Geometry check sheet. Reference: the model listing, model coordinates, mm. Face numbers are marked on the shaded views. A direction names the side the tool comes from. Give positions to 0.01 mm unless a question says otherwise; leave off trailing zeros. Loops run counter-clockwise (first coordinate to the right, second up) from the corner with the lowest first, then second, coordinate; pieces in that order, holes last. Notation, with made-up numbers: (48.5, 48.5) -> (57.5, 48.5) arc R13 cw to (57.5, 69.5) -> close; hole circle Ø1 at (75.5, 88.25). An arc over 180 degrees is marked (long way). Answer as a JSON object with one key per item and string values.
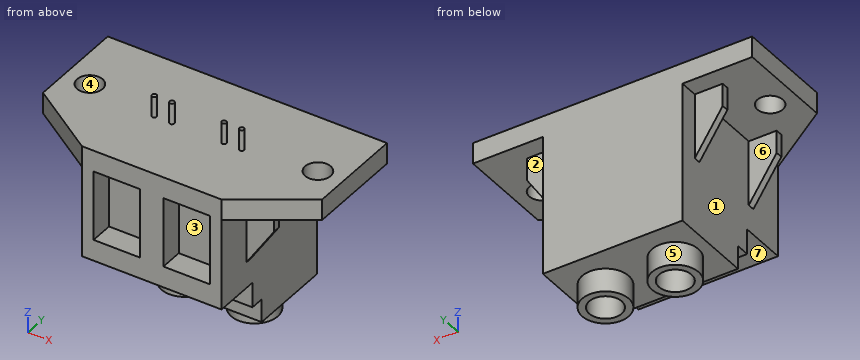
from build123d import *

# Parameters (mm, degrees)
SKETCH_1_R           = 2.75
EXTRUDE_1_DEPTH      = 4.5
EXTRUDE_2_DEPTH      = 15
EXTRUDE_2_DEPTH_BACK = 15
SKETCH_3_R           = 5
SKETCH_3_R_2         = 3.5
EXTRUDE_3_DEPTH      = 5
SKETCH_4_W           = 10
SKETCH_4_H           = 15
CUT_EXTRUDE_1_DEPTH  = 5
SKETCH_5_R           = 0.5
EXTRUDE_4_DEPTH      = 4.5
SKETCH_6_W           = 6
SKETCH_6_H           = 1.5
EXTRUDE_5_DEPTH      = 14
CUT_EXTRUDE_2_DEPTH  = 20


with BuildPart() as part:
    # Эскиз1 → Вытянуть1 (new body)
    with BuildSketch(Plane.XY):
        Polygon((-15, -16.9), (-30, -6.9), (-30, 14.1), (30, 14.1), (30, -6.9), (15, -16.9), align=None)
        with Locations((-24.5, 0)):
            Circle(SKETCH_1_R, mode=Mode.SUBTRACT)
        with Locations((24.5, 0)):
            Circle(SKETCH_1_R, mode=Mode.SUBTRACT)
    extrude(amount=EXTRUDE_1_DEPTH)

    # Эскиз2 → Вытянуть2 (add, two sides: drawn at the far end of the back side and taken through both)
    with BuildSketch(Plane(origin=(0, 0, 0), x_dir=(0, 0, -1), z_dir=(1, 0, 0)).offset(-EXTRUDE_2_DEPTH_BACK)):
        Polygon((0, -16.9), (19.60451018, -16.9), (19.60451018, -6.9), (25, -6.9), (25, -3.9), (30, -3.9), (30, 14.1), (0, 14.1), align=None)
    extrude(amount=EXTRUDE_2_DEPTH + EXTRUDE_2_DEPTH_BACK)

    # Эскиз3 → Вытянуть3 (add)
    # profile 1 of 2: a face of its own
    with BuildSketch(Plane(origin=(0, 0, -30), x_dir=(-1, 0, 0), z_dir=(0, 0, -1))):
        with Locations(Location((-7.5, 5.1, 0), (0, 0, 180))):
            Circle(SKETCH_3_R)
        with Locations((-7.5, 5.1)):
            Circle(SKETCH_3_R_2, mode=Mode.SUBTRACT)
    # profile 2 of 2: a face of its own
    with BuildSketch(Plane(origin=(0, 0, -30), x_dir=(-1, 0, 0), z_dir=(0, 0, -1))):
        with Locations(Location((7.5, 5.1, 0), (0, 0, 180))):
            Circle(SKETCH_3_R)
        with Locations((7.5, 5.1)):
            Circle(SKETCH_3_R_2, mode=Mode.SUBTRACT)
    extrude(amount=EXTRUDE_3_DEPTH)

    # Эскиз4 → Вырез-Вытянуть1 (cut)
    with BuildSketch(Plane.XZ.offset(16.9)):
        with Locations((7.5, -7.55225509)):
            Rectangle(SKETCH_4_W, SKETCH_4_H)
        with Locations((-7.5, -7.55225509)):
            Rectangle(SKETCH_4_W, SKETCH_4_H)
    extrude(amount=-CUT_EXTRUDE_1_DEPTH, mode=Mode.SUBTRACT)

    # Эскиз5 → Вытянуть4 (add)
    with BuildSketch(Plane.XY.offset(4.5)):
        with Locations(Location((-9.4, -1.9, 0), (0, 0, 180))):
            Circle(SKETCH_5_R)
        with Locations(Location((-5.6, -1.9, 0), (0, 0, 180))):
            Circle(SKETCH_5_R)
        with Locations(Location((5.6, -1.9, 0), (0, 0, 180))):
            Circle(SKETCH_5_R)
        with Locations(Location((9.4, -1.9, 0), (0, 0, 180))):
            Circle(SKETCH_5_R)
    extrude(amount=EXTRUDE_4_DEPTH)

    # Эскиз6 → Вытянуть5 (add)
    with BuildSketch(Plane(origin=(0, 0, 0), x_dir=(-1, 0, 0), z_dir=(0, 0, -1))):
        with Locations((-18, -8.15)):
            Rectangle(SKETCH_6_W, SKETCH_6_H)
        with Locations((-18, 9.35)):
            Rectangle(SKETCH_6_W, SKETCH_6_H)
        with Locations((18, 9.35)):
            Rectangle(SKETCH_6_W, SKETCH_6_H)
        with Locations((18, -8.15)):
            Rectangle(SKETCH_6_W, SKETCH_6_H)
    extrude(amount=EXTRUDE_5_DEPTH)

    # Эскиз7 → Вырез-Вытянуть2 (cut)
    with BuildSketch(Plane.XZ.offset(8.9)):
        Polygon((15, -14), (22.174858564, -3.085279584), (22.174858564, -17.29993251), align=None)
        Polygon((-22.174858564, -17.29993251), (-15, -14), (-22.174858564, -3.085279584), align=None)
    extrude(amount=-CUT_EXTRUDE_2_DEPTH, mode=Mode.SUBTRACT)


solid = part.part
1) Material ranges on line 1 along X through (y, z) = (-15, -5); line 2 along Y through (x, z) = (15.5, -13); line 3 along Z through (x, y) = (8.5, -12), recorded low to high. Write a range as from..to.
Geometry check:
{"line 1": "x = -15..-12.5, -2.5..2.5, 12.5..15", "line 2": "y = -8.9..-7.4, 8.6..10.1", "line 3": "z = -19.6..-15.05, -0.05..4.5"}
2) Section check C-C on z = -12. Record the cut outline in (x, y).
Geometry check:
{"outline": "(-16.31, -8.9) -> (-15, -8.9) -> (-15, -16.9) -> (-12.5, -16.9) -> (-12.5, -11.9) -> (-2.5, -11.9) -> (-2.5, -16.9) -> (2.5, -16.9) -> (2.5, -11.9) -> (12.5, -11.9) -> (12.5, -16.9) -> (15, -16.9) -> (15, -8.9) -> (16.31, -8.9) -> (16.31, -7.4) -> (15, -7.4) -> (15, 8.6) -> (16.31, 8.6) -> (16.31, 10.1) -> (15, 10.1) -> (15, 14.1) -> (-15, 14.1) -> (-15, 10.1) -> (-16.31, 10.1) -> (-16.31, 8.6) -> (-15, 8.6) -> (-15, -7.4) -> (-16.31, -7.4) -> close"}
3) Section check D-D on x = 24.5. Record the cut outline in (y, z).
Geometry check:
{"outline": "(-10.57, 0) -> (-2.75, 0) -> (-2.75, 4.5) -> (-10.57, 4.5) -> close; (2.75, 0) -> (14.1, 0) -> (14.1, 4.5) -> (2.75, 4.5) -> close"}
4) Section check A-A on y = 5.1. Record the cut outline in (x, z).
Geometry check:
{"outline": "(-30, 0) -> (-15, 0) -> (-15, -30) -> (-12.5, -30) -> (-12.5, -35) -> (-11, -35) -> (-11, -30) -> (-4, -30) -> (-4, -35) -> (-2.5, -35) -> (-2.5, -30) -> (2.5, -30) -> (2.5, -35) -> (4, -35) -> (4, -30) -> (11, -30) -> (11, -35) -> (12.5, -35) -> (12.5, -30) -> (15, -30) -> (15, 0) -> (30, 0) -> (30, 4.5) -> (-30, 4.5) -> close"}
5) Section check B-B on x = 0.5. Record the cut outline in (y, z), plus the area to 3 significant figures.
Geometry check:
{"outline": "(-16.9, -19.6) -> (-6.9, -19.6) -> (-6.9, -25) -> (-3.9, -25) -> (-3.9, -30) -> (14.1, -30) -> (14.1, 4.5) -> (-16.9, 4.5) -> close", "area": "951 mm2"}
6) Tool access check on the marked faces 5, 6 and 7. Record the directions out of +Z, -Z, +X, -X, +Y, -Y that give a thin tool (end or side, any length) a straight path to the whole face; none if there is none.
Geometry check:
{"face 5": "-Z", "face 6": "-Z, -X", "face 7": "-Z, +X, -X, -Y"}
7) Depth check by flat-ended pin: P1, Ø6, axis at y = -9, z = -10, coming from the +X side; P2, Ø3, axis at x = -15.5, y = 0.5, coming from the +Z side; P3, Ø1.6, axis at y = -8, z = -2.5, coming from the -X side. Enter the tip coordinate at first touch or a pass-through.
Geometry check:
{"P1": "stops at x = 19.6", "P2": "stops at z = 4.5", "P3": "stops at x = -21"}
8) Draft check along X on the marked faces 1, 2, 3 and 4. Enter one of: pulls with the +X half, pulls with the -X half, needs draft (parallel to the pull), parting line crosses it, or undercut.
Geometry check:
{"face 1": "pulls with the -X half", "face 2": "needs draft", "face 3": "undercut", "face 4": "undercut"}
